from build123d import *

# Parameters (mm, degrees)
F1_DEPTH = 1.524
F3_DEPTH = 1.524
F4_DEPTH = 25.4


with BuildPart() as f1:
    # F0 (on Front) → F1 (new body)
    with BuildSketch(Plane.XZ):
        with BuildLine():
            ThreePointArc((-16.676399, 24.306558), (-12.453754, 21.27727), (-8.231109, 24.306558))
            ThreePointArc((-8.231109, 24.306558), (-7.830954, 26.73827), (-8.231109, 29.169981))
            ThreePointArc((-8.231109, 29.169981), (-12.453754, 32.19927), (-16.676399, 29.169981))
            ThreePointArc((-16.676399, 29.169981), (-17.076554, 26.73827), (-16.676399, 24.306558))
        make_face()
        with BuildLine():
            ThreePointArc((-15.593669, 28.803722), (-12.453754, 31.05627), (-9.313838, 28.803722))
            ThreePointArc((-9.313838, 28.803722), (-8.973954, 26.73827), (-9.313838, 24.672818))
            ThreePointArc((-9.313838, 24.672818), (-12.453754, 22.42027), (-15.593669, 24.672818))
            ThreePointArc((-15.593669, 24.672818), (-15.933554, 26.73827), (-15.593669, 28.803722))
        make_face(mode=Mode.SUBTRACT)
    extrude(amount=F1_DEPTH)

    # F2 (on face) → F3 (join)
    with BuildSketch(Plane.XZ.offset(1.524)):
        with BuildLine():
            ThreePointArc((-9.313838, 24.672818), (-9.282874, 24.76672), (-9.253354, 24.861087))
            Line((-9.253354, 24.861087), (-9.253354, 26.73827))
            Line((-9.253354, 26.73827), (-12.453754, 26.73827))
            Line((-12.453754, 26.73827), (-12.453754, 25.59527))
            Line((-12.453754, 25.59527), (-10.396354, 25.59527))
            Line((-10.396354, 25.59527), (-10.396354, 23.136058))
            ThreePointArc((-10.396354, 23.136058), (-9.743877, 23.826094), (-9.313838, 24.672818))
        make_face()
    extrude(amount=-F3_DEPTH)

    # F2 (on face) → F4 (cut)
    with BuildSketch(Plane.XZ.offset(1.524)):
        with BuildLine():
            Line((-9.253354, 24.861087), (-9.253354, 22.631983))
            ThreePointArc((-9.253354, 22.631983), (-8.64896, 23.412333), (-8.231109, 24.306558))
            ThreePointArc((-8.231109, 24.306558), (-7.830954, 26.73827), (-8.231109, 29.169981))
            ThreePointArc((-8.231109, 29.169981), (-8.650336, 30.066457), (-9.257028, 30.848342))
            Line((-9.257028, 30.848342), (-9.967955, 29.934294))
            ThreePointArc((-9.967955, 29.934294), (-9.584657, 29.401546), (-9.313838, 28.803722))
            ThreePointArc((-9.313838, 28.803722), (-8.974712, 26.837143), (-9.253354, 24.861087))
        make_face()
    extrude(amount=-F4_DEPTH, mode=Mode.SUBTRACT)


solid = f1.part
Input: part model. Units: mm. Frame: model coordinates. A direction names the side the tool comes from. Coordinates: 2 decimals unless noted, no trailing zeros. Loops run counter-clockwise (first coordinate to the right, second up) from the corner with the lowest first, then second, coordinate; pieces in that order, holes last. Notation, with made-up numbers: (0, 44) -> (52, 44) arc R14 ccw to (52, 61) -> close; hole circle Ø1 at (20, 13). An arc over 180 degrees is marked (long way). Write item = value, one per line. Start each with the question number.
Item 1: Reachability of faces 1 (the face through (-9.253, -1, 25)), 2 (the face through (-11, -1, 26.738)), 3 (the face through (-11, -1, 25.595)) from +Z, -Z, +X, -X, +Y, -Y: full face, straight path, thin tool, end or side. Return the list, or none.
Item 2: Cut plane B-B, the plane z = 24.5. Return loops of the section in (x, y), plus the area to 3 significant figures.
Item 3: Mould query, pull axis X, two halves, no side actions, for faces 4 (the face through (-13.154, -0.751, 30.981)), 5 (the face through (-17.076, -0.751, 26.773)), 6 (the face through (-12, 0, 26)). Classes: pulls with the +X half, pulls with the -X half, needs draft (parallel to the pull), parting line crosses it, or undercut.
Item 4: Cut plane C-C, the plane y = -1.25. Return loops of the section in (x, z), plus the area to 3 significant figures.
Item 5: Material intervals for line 1 (Z direction, x = -12.5, y = -1.2); line 2 (X direction, y = -1.35, z = 24.75); line 3 (Z direction, x = -10.5, y = -1), sorted ascending.
Item 6: First-contact query: P1, Ø1.5, axis at x = -13.5, z = 23.5, coming from the -Y side; P2, Ø0.5, axis at y = -0.5, z = 24.5, coming from the -X side. Flat tips, straight axial feed; report the tip coordinate or a pass-through.
Item 7: Cut plane D-D, the plane x = -11.25. Return loops of the section in (y, z), plus the area to 3 significant figures.
Item 8: Cut plane A-A, the plane x = -9.5. Return loops of the section in (y, z).
Ans:
q1.face_1 = +Z, -Z, +X, +Y, -Y
q1.face_2 = +X, +Y, -Y
q1.face_3 = +Y, -Y
q2.outline = (-16.74, -1.52) -> (-15.53, -1.52) -> (-15.53, 0) -> (-16.74, 0) -> close; (-10.4, -1.52) -> (-9.25, -1.52) -> (-9.25, 0) -> (-10.4, 0) -> close
q2.area = 3.58 mm²
q3.face_4 = undercut
q3.face_5 = pulls with the -X half
q3.face_6 = needs draft
q4.outline = (-16.68, 24.31) arc R4.46 ccw to (-9.25, 22.63) -> (-9.25, 26.74) -> (-12.45, 26.74) -> (-12.45, 25.6) -> (-10.4, 25.6) -> (-10.4, 23.14) arc R3.31 cw to (-15.59, 24.67) arc R6.45 cw to (-15.59, 28.8) arc R3.31 cw to (-9.97, 29.93) -> (-9.26, 30.85) arc R4.46 ccw to (-16.68, 29.17) arc R7.59 ccw to start
q4.area = 30.0 mm²
q5.line_1 = 21.28 to 22.42, 31.06 to 32.2
q5.line_2 = -16.81 to -15.62, -10.4 to -9.25
q5.line_3 = 21.73 to 23.06, 25.6 to 26.74, 30.42 to 31.75
q6.P1 = through
q6.P2 = -16.81
q7.outline = (-1.52, 21.44) -> (0, 21.44) -> (0, 22.65) -> (-1.52, 22.65) -> close; (-1.52, 25.6) -> (0, 25.6) -> (0, 26.74) -> (-1.52, 26.74) -> close; (-1.52, 30.83) -> (0, 30.83) -> (0, 32.03) -> (-1.52, 32.03) -> close
q7.area = 5.41 mm²
q8.outline = (-1.52, 22.4) -> (0, 22.4) -> (0, 26.74) -> (-1.52, 26.74) -> close; (-1.52, 30.54) -> (0, 30.54) -> (0, 31.08) -> (-1.52, 31.08) -> close
